```python
from build123d import *

# Parameters (mm, degrees)
SKETCH2_R           = 1.6
BOSS_EXTRUDE1_DEPTH = 1.2


with BuildPart() as part:
    # Sketch2 → Boss-Extrude1 (new body)
    with BuildSketch(Plane.XY.offset(9.801785136)):
        Polygon((-28, -37.413217807), (-32, -33.413217807), (-32, 11.586782193), (32, 11.586782193), (32.017485427, -33.413217807), (28.017485427, -37.413217807), align=None)
        with Locations((-15, 5.74456922)):
            Circle(SKETCH2_R, mode=Mode.SUBTRACT)
        with Locations((15, 5.74456922)):
            Circle(SKETCH2_R, mode=Mode.SUBTRACT)
        with Locations((-15, -30.25543078)):
            Circle(SKETCH2_R, mode=Mode.SUBTRACT)
        with Locations((15, -30.25543078)):
            Circle(SKETCH2_R, mode=Mode.SUBTRACT)
    extrude(amount=BOSS_EXTRUDE1_DEPTH)


solid = part.part
```
Check sheet for the modelled part. Datum: model origin and axes. Units: mm. Round coordinates to 2 decimals unless told otherwise and drop trailing zeros. Order: outer loops, then holes, each group sorted by start corner. A loop starts at its lowest first (then second) coordinate and runs counter-clockwise, first axis right, second up. Notation, with made-up numbers: (7.5, 89) -> (44.5, 89) arc R23 ccw to (44.5, 97) -> close; hole circle Ø6 at (-17.75, -4.75). An arc over 180 degrees is marked (long way). Use CSV: the item, a comma, the result in double quotes.
(1) Depth check by flat-ended pin: pin 1 (0.6 mm diameter, centred on y = -20, z = 10.5, fed in from +X). Enter the tip coordinate at first touch or a pass-through.
Worked out:
pin 1,"x = 32.01"
(2) Cross-section at B-B (z = 10.4). Record the boundary of the cut face in (x, y).
Worked out:
outline,"(-32, -33.41) -> (-28, -37.41) -> (28.02, -37.41) -> (32.02, -33.41) -> (32, 11.59) -> (-32, 11.59) -> close; hole circle Ø3.2 at (-15, -30.26); hole circle Ø3.2 at (-15, 5.74); hole circle Ø3.2 at (15, -30.26); hole circle Ø3.2 at (15, 5.74)"
(3) Cross-section at A-A (x = -15). Record the boundary of the cut face in (y, z), and give its area (3 significant figures).
Worked out:
outline,"(-37.41, 9.8) -> (-31.86, 9.8) -> (-31.86, 11) -> (-37.41, 11) -> close; (-28.66, 9.8) -> (4.14, 9.8) -> (4.14, 11) -> (-28.66, 11) -> close; (7.34, 9.8) -> (11.59, 9.8) -> (11.59, 11) -> (7.34, 11) -> close"
area,"51.1 mm²"
(4) Draft check along X on faces 1 (the face through (0, -13, 9.802)), 2 (the face through (-29.972, -35.441, 10.393)), 3 (the face through (13.4, 5.8, 10.4)). Enter one of: pulls with the +X half, pulls with the -X half, needs draft (parallel to the pull), parting line crosses it, or undercut.
Worked out:
face 1,"needs draft"
face 2,"pulls with the -X half"
face 3,"undercut"
(5) Material ranges on line 1 along Y through (x, z) = (-15, 10.4); line 2 along X through (y, z) = (-29, 9.9); line 3 along X through (y, z) = (-1, 10.85), recorded low to high. Write a range as from..to.
Worked out:
line 1,"-37.41..-31.86, -28.66..4.14, 7.34..11.59"
line 2,"-32..-15.99, -14.01..14.01, 15.99..32.02"
line 3,"-32..32"
